```python
from build123d import *

# Parameters (mm, degrees)
CROQUIS1_W              = 23.5
CROQUIS1_H              = 10
CROQUIS1_W_2            = 7
CROQUIS1_R              = 1.5
SALIENTE_EXTRUIR1_DEPTH = 5
CROQUIS1_3_W            = 7
CROQUIS1_3_H            = 10
CROQUIS1_3_R            = 1.5
SALIENTE_EXTRUIR2_DEPTH = 5


with BuildPart() as part:
    # Croquis1 → Saliente-Extruir1 (new body)
    with BuildSketch(Plane(origin=(0, 0, 0), x_dir=(1, 0, 0), z_dir=(0, 1, 0))):
        Rectangle(CROQUIS1_W, CROQUIS1_H)
        with Locations((-15.25, 0)):
            Rectangle(CROQUIS1_W_2, CROQUIS1_H)
        with Locations((-15, 0)):
            Circle(CROQUIS1_R, mode=Mode.SUBTRACT)
        with Locations((-15, 0)):
            Circle(CROQUIS1_R)
        with Locations((15.25, 0)):
            Rectangle(CROQUIS1_W_2, CROQUIS1_H)
        with Locations((15, 0)):
            Circle(CROQUIS1_R, mode=Mode.SUBTRACT)
        with Locations((15, 0)):
            Circle(CROQUIS1_R)
    extrude(amount=SALIENTE_EXTRUIR1_DEPTH)

    # Croquis1_3 → Saliente-Extruir2 (add)
    with BuildSketch(Plane(origin=(0, 0, 0), x_dir=(1, 0, 0), z_dir=(0, 1, 0))):
        with Locations((-15.25, 0)):
            Rectangle(CROQUIS1_3_W, CROQUIS1_3_H)
        with Locations(Location((-15, 0, 0), (0, 0, 270))):
            Circle(CROQUIS1_3_R, mode=Mode.SUBTRACT)
        with Locations((15.25, 0)):
            Rectangle(CROQUIS1_3_W, CROQUIS1_3_H)
        with Locations(Location((15, 0, 0), (0, 0, 270))):
            Circle(CROQUIS1_3_R, mode=Mode.SUBTRACT)
    extrude(amount=-SALIENTE_EXTRUIR2_DEPTH)


solid = part.part
```
Here's how the part is built. I have some questions about the finished solid (model axes, mm). A direction names the side the tool comes from. Give positions to 0.01 mm unless a question says otherwise; leave off trailing zeros. Order: outer loops, then holes, each group sorted by start corner. A loop starts at its lowest first (then second) coordinate and runs counter-clockwise, first axis right, second up. Notation, with made-up numbers: M 6.5,39.25 L 14.5,39.25 A20 ccw 14.5,68.25 Z; hole C 46.5,83 d4. An arc over 180 degrees is marked long. Use a Markdown table: item, result. Add a question column.
1. On a 3-axis mill with a long thin cutter (end or side, diameter ignored), from which of +Z, -Z, +X, -X, +Y, -Y can I reach the whole of each face in a straight line? I mean faces 1 (the flat face through (-11.75, -2, 0)), 2 (the flat face through (15, 0, 0)), 3 (the flat face through (0, 5, 0)). Say none if no direction works.
2. Suppose I cut it at C-C (x = -15). List the corners of the cut face in (y, z) for me, and give its area (3 significant figures).
3. For pin 1 Ø2.5 at (x, z) = (-15.5, 0.5) entering from -Y, with a flat end and sliding along its axis, tell me the tip position at first contact or that it passes through.
4. If we mould it in two halves opening along Z, with no side actions, what happens to faces 4 (the cylindrical face through (-14.55, -2.46, 1.43)), 5 (the flat face through (0, 1, -5)), 6 (the flat face through (-18.75, 0, 0)), 7 (the flat face through (-15, 0, 0))? For each: +Z half, -Z half, draft (parallel to the pull), parting line (faces both ways), or undercut.
5. Suppose I cut it at A-A (y = -2). List the corners of the cut face in (x, z) for me.
6. Suppose I cut it at D-D (z = 0). List the corners of the cut face in (x, y) for me, and give its area (4 significant figures).
7. Suppose I cut it at B-B (z = 3.5). List the corners of the cut face in (x, y) for me, and give its area (4 significant figures).
8. I need wall thicknesses on probe 1 along X at (y, z) = (-1.4, 0); probe 2 along X at (y, z) = (-2, 2.25); probe 3 along Y at (x, z) = (-0.5, 4.75). Which ranges of each line are inside material? Lowest first, please. Write a range as from..to.
Results list:
| question | item | result |
|---|---|---|
| 1 | face 1 | +Z, -Z, -Y |
| 1 | face 2 | -Y |
| 1 | face 3 | +Z, -Z, +X, -X, +Y |
| 2 | outline | M -5,-5 L 5,-5 L 5,5 L -5,5 L -5,1.5 L 0,1.5 L 0,-1.5 L -5,-1.5 Z |
| 2 | area | 85.0 mm² |
| 3 | pin 1 | stops at y = -5 |
| 4 | face 4 | undercut |
| 4 | face 5 | -Z half |
| 4 | face 6 | draft |
| 4 | face 7 | undercut |
| 5 | outline | M -18.75,-5 L -11.75,-5 L -11.75,5 L -18.75,5 Z; M 11.75,-5 L 18.75,-5 L 18.75,5 L 11.75,5 Z; hole C -15,0 d3; hole C 15,0 d3 |
| 6 | outline | M -18.75,-5 L -16.5,-5 L -16.5,0 L -13.5,0 L -13.5,-5 L -11.75,-5 L -11.75,0 L 11.75,0 L 11.75,-5 L 13.5,-5 L 13.5,0 L 16.5,0 L 16.5,-5 L 18.75,-5 L 18.75,5 L -18.75,5 Z |
| 6 | area | 227.5 mm² |
| 7 | outline | M -18.75,-5 L -11.75,-5 L -11.75,0 L 11.75,0 L 11.75,-5 L 18.75,-5 L 18.75,5 L -18.75,5 Z |
| 7 | area | 257.5 mm² |
| 8 | probe 1 | x = -18.75..-16.5, -13.5..-11.75, 11.75..13.5, 16.5..18.75 |
| 8 | probe 2 | x = -18.75..-11.75, 11.75..18.75 |
| 8 | probe 3 | y = 0..5 |
